Design review of the part shown in the three views and the two pictorial views. Dimensions are in mm from the part's minimum x, y and z. A direction names the side the tool comes from. Round coordinates to 2 decimals unless told otherwise and drop trailing zeros. Order: outer loops, then holes, each group sorted by start corner. A loop starts at its lowest first (then second) coordinate and runs counter-clockwise, first axis right, second up. Notation, with made-up numbers: M 59.5,-4.75 L 99.5,-4.75 A20 cw 99.5,20.25 Z; hole C 60.25,-4 d4. An arc over 180 degrees is marked long. Write item = value, one per line. Start each with the question number.
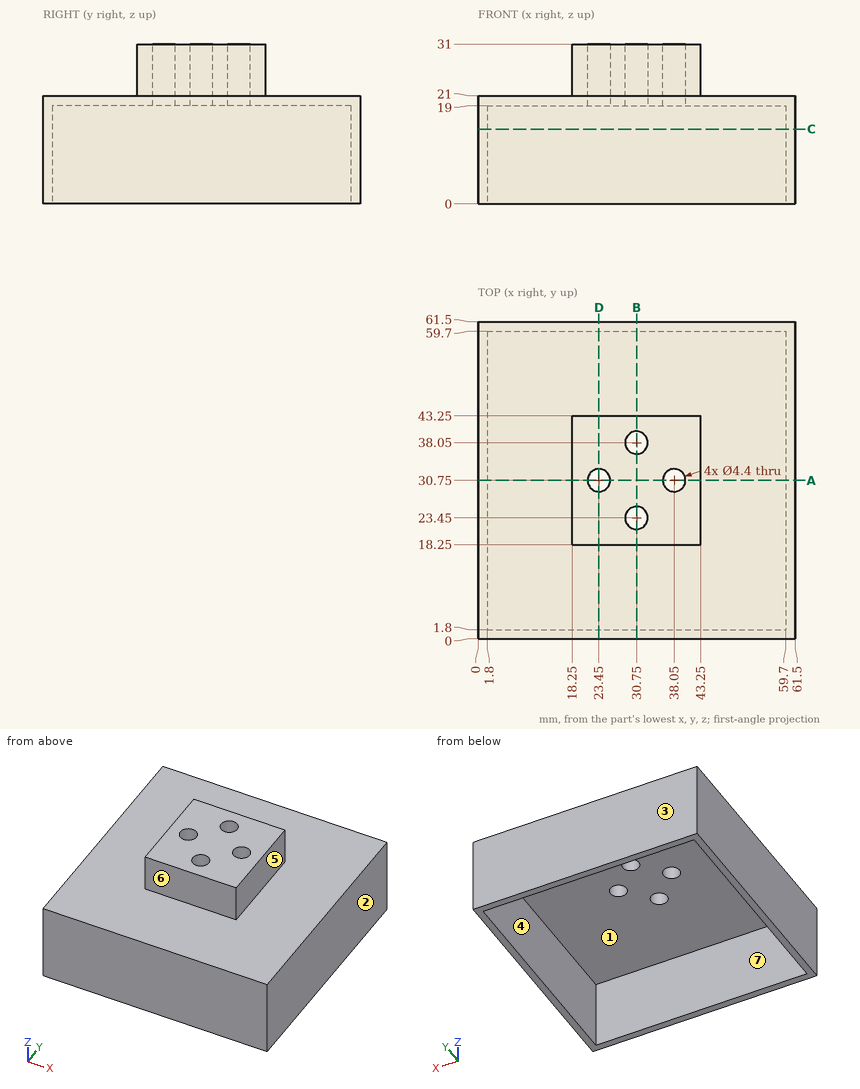
(1) For line 1 along X through (y, z) = (36.5, 4.5); line 2 along Y through (x, z) = (23.45, 25.5), list the stretches that pass through material, from the lowest coordinate up.
(2) We need section C-C, the plane z = 14.5. Write out the cut boundary in (x, y), then the cut area to 3 significant figures.
(3) Draft analysis for pull direction X (two halves, no side actions). For the marked faces 1, 2, 3 and 4, state which applies: released by +X, released by -X, zero draft, split by the parting line, or undercut.
(4) Insertion check: pin 1 (8 mm diameter, centred on y = 30, z = 25.5, fed in from -X); pin 2 (2 mm diameter, centred on x = 32, z = 25, fed in from +Y); pin 3 (5 mm diameter, centred on x = 30, z = 28, fed in from -Y). Each pin has a flat end and moves straight along its axis. Give the tip position at first contact, or say it passes through.
(5) We need section D-D, the plane x = 23.45. Write out the cut boundary in (y, z).
(6) We need section A-A, the plane y = 30.75. Write out the cut boundary in (x, z), then the cut area to 3 significant figures.
(7) For the marked faces 5, 6 and 7, list the 3-axis set-ups (+Z, -Z, +X, -X, +Y, -Y) from which the entire face can be reached by the end or side of a thin tool; tool diameter is ignored.
Values:
q1.line_1 = 0 to 1.8, 59.7 to 61.5
q1.line_2 = 18.25 to 28.55, 32.95 to 43.25
q2.outline = M 0,0 L 61.5,0 L 61.5,61.5 L 0,61.5 Z; hole M 1.8,1.8 L 59.7,1.8 L 59.7,59.7 L 1.8,59.7 Z
q2.area = 430 mm²
q3.face_1 = undercut
q3.face_2 = released by +X
q3.face_3 = zero draft
q3.face_4 = undercut
q4.pin_1 = 18.25
q4.pin_2 = 43.25
q4.pin_3 = 18.25
q5.outline = M 0,0 L 1.8,0 L 1.8,19 L 28.55,19 L 28.55,31 L 18.25,31 L 18.25,21 L 0,21 Z; M 32.95,19 L 59.7,19 L 59.7,0 L 61.5,0 L 61.5,21 L 43.25,21 L 43.25,31 L 32.95,31 Z
q6.outline = M 0,0 L 1.8,0 L 1.8,19 L 21.25,19 L 21.25,31 L 18.25,31 L 18.25,21 L 0,21 Z; M 25.65,19 L 35.85,19 L 35.85,31 L 25.65,31 Z; M 40.25,19 L 59.7,19 L 59.7,0 L 61.5,0 L 61.5,21 L 43.25,21 L 43.25,31 L 40.25,31 Z
q6.area = 336 mm²
q7.face_5 = +Z, +X, +Y, -Y
q7.face_6 = +Z, +X, -X, -Y
q7.face_7 = -Z
